Can you work these out from the model? Positions are in its coordinate system, mm. Face numbers are marked on the shaded views. A direction names the side the tool comes from. Give positions to 0.01 mm unless a question says otherwise; leave off trailing zeros. Loops run counter-clockwise (first coordinate to the right, second up) from the corner with the lowest first, then second, coordinate; pieces in that order, holes last. Notation, with made-up numbers: (78.5, 8.5) - (105.5, 8.5) arc R17 ccw to (105.5, 27.5) - close; hole circle Ø11 at (53.5, -25.5). An arc over 180 degrees is marked (long way). Use a Markdown table: item, result. Add a question column.
```python
from build123d import *

# Parameters (mm, degrees)
SKETCH1_R           = 6
BOSS_EXTRUDE1_DEPTH = 150
CUT_EXTRUDE1_DEPTH  = 150
CUT_EXTRUDE2_DEPTH  = 150
SKETCH6_R           = 2.5
CUT_EXTRUDE3_DEPTH  = 150


with BuildPart() as part:
    # Sketch1 → Boss-Extrude1 (new body)
    with BuildSketch(Plane(origin=(0, 0, 0), x_dir=(0, 0, -1), z_dir=(1, 0, 0))):
        with BuildLine():
            Line((-10.816901408, 22.056338028), (-10.816901408, -15.943661972))
            Line((-10.816901408, -15.943661972), (13.183098592, -15.943661972))
            Line((13.183098592, -15.943661972), (13.183098592, 22.056338028))
            ThreePointArc((13.183098592, 22.056338028), (1.183098592, 34.056338028), (-10.816901408, 22.056338028))
        make_face()
        with Locations((1.183098592, 2.056338028)):
            Circle(SKETCH1_R, mode=Mode.SUBTRACT)
    extrude(amount=-BOSS_EXTRUDE1_DEPTH)

    # Sketch3 → Cut-Extrude1 (cut)
    with BuildSketch(Plane(origin=(0, 0, -13.183098592), x_dir=(-1, 0, 0), z_dir=(0, 0, -1))):
        with BuildLine():
            Line((5, 34.056338028), (5, -6.943661972))
            ThreePointArc((5, -6.943661972), (6.171572875, -9.772089097), (9, -10.943661972))
            Line((9, -10.943661972), (150, -10.943661972))
            Line((150, -10.943661972), (150, 34.056338028))
            Line((150, 34.056338028), (5, 34.056338028))
        make_face()
    extrude(amount=-CUT_EXTRUDE1_DEPTH, mode=Mode.SUBTRACT)

    # Sketch4 → Cut-Extrude2 (cut)
    with BuildSketch(Plane(origin=(0, 0, -13.183098592), x_dir=(-1, 0, 0), z_dir=(0, 0, -1))):
        Polygon((146.731773505, -10.943661972), (150, -12.910119048), (150, -10.943661972), align=None)
        with BuildLine():
            Line((0, -6.943663252), (0, -15.943661972))
            Line((0, -15.943661972), (8.999719534, -15.943661972))
            ThreePointArc((8.999719534, -15.943661972), (2.635939888, -13.307524671), (0, -6.943663252))
        make_face()
    extrude(amount=-CUT_EXTRUDE2_DEPTH, mode=Mode.SUBTRACT)

    # Sketch6 → Cut-Extrude3 (cut)
    with BuildSketch(Plane(origin=(0, -10.943661972, 0), x_dir=(1, 0, 0), z_dir=(0, 1, 0))):
        with Locations(Location((-70, 1.183098592, 0), (0, 0, 180))):
            Circle(SKETCH6_R)
    extrude(amount=-CUT_EXTRUDE3_DEPTH, mode=Mode.SUBTRACT)


solid = part.part
```
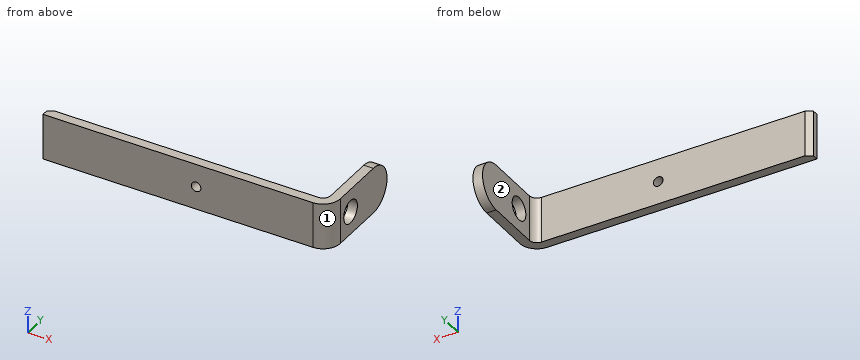
1. Suppose I cut it at D-D (y = 18.5). List the corners of the cut face in (x, z) for me.
2. Will these pins go through, and if not, where does the flat tip stop? P1, Ø4, axis at x = -70, z = -1.18, coming from the -Y side; P2, Ø12, axis at x = -65.5, z = 2, coming from the +Y side; P3, Ø14, axis at y = 2.06, z = -1.18, coming from the -X side; P4, Ø2, axis at y = -8.5, z = -5.5, coming from the +X side.
3. Please list where these lines run through material, in increasing order: line 1 along X through (y, z) = (26, -7.5); line 2 along Y through (x, z) = (-85, 0.25); line 3 along X through (y, z) = (-11.5, -7). Write a range as [from, to].
4. On a 3-axis mill with a long thin cutter (end or side, diameter ignored), from which of +Z, -Z, +X, -X, +Y, -Y can I reach the whole of each face in a straight line? I mean the marked faces 1 and 2. Say none if no direction works.
5. Suppose I cut it at A-A (x = -70). List the corners of the cut face in (y, z) for me.
6. Suppose I cut it at B-B (y = 5.5). List the corners of the cut face in (x, z) for me, and give its area (3 significant figures).
7. Suppose I cut it at C-C (z = 6.75). List the corners of the cut face in (x, y) for me, and give its area (3 significant figures).
Results below:
| question | item | result |
|---|---|---|
| 1 | outline | (-5, -13.18) - (0, -13.18) - (0, 10.82) - (-5, 10.82) - close |
| 2 | P1 | through |
| 2 | P2 | y = -10.94 |
| 2 | P3 | x = -5 |
| 2 | P4 | x = -0.02 |
| 3 | line 1 | [-5, 0] |
| 3 | line 2 | [-15.94, -10.94] |
| 3 | line 3 | [-147.66, -1.24] |
| 4 | face 1 | +Z, -Z, +X, -Y |
| 4 | face 2 | +Z, -Z, -X, +Y |
| 5 | outline | (-15.94, -13.18) - (-10.94, -13.18) - (-10.94, -3.68) - (-15.94, -3.68) - close; (-15.94, 1.32) - (-10.94, 1.32) - (-10.94, 10.82) - (-15.94, 10.82) - close |
| 6 | outline | (-5, -13.18) - (0, -13.18) - (0, -6.1) - (-5, -6.1) - close; (-5, 3.73) - (0, 3.73) - (0, 10.82) - (-5, 10.82) - close |
| 6 | area | 70.9 mm² |
| 7 | outline | (-150, -15.94) - (-9, -15.94) arc R9 ccw to (0, -6.94) - (0, 31.06) - (-5, 31.06) - (-5, -6.94) arc R4 cw to (-9, -10.94) - (-146.73, -10.94) - (-150, -12.91) - close |
| 7 | area | 943 mm² |
